Autodesk Inventor part; units mm, degrees
ref_plane "Work Plane1" through (-65, 0, -15) normal (0, 0, 1) x (1, 0, 0)
ref_plane "YZ Plane" through (0, 0, 0) normal (1, 0, 0) x (0, 1, 0)
ref_plane "XZ Plane" through (0, 0, 0) normal (0, 1, 0) x (-1, 0, 0)
sketch "Sketch1" plane through (0, 0, 0) normal (0, 1, 0) x (-1, 0, 0)
  line L0 (0, 0) -> (65, 0)
  line L1 (65, 0) -> (65, -30)
  line L2 (65, -30) -> (0, -30)
  line L3 (0, -30) -> (0, 0)
  dimension "d0" = 65
  dimension "d1" = 30
extrude "Extrusion1" add sketch "Sketch1" along normal blind 20
sketch "Sketch2" plane through (-65, 0, 0) normal (0, 0, 1) x (1, 0, 0)
  line L0 (5, 18) -> (15, 18)
  line L1 (15, 18) -> (15, 13)
  line L2 (15, 13) -> (5, 13)
  line L3 (5, 13) -> (5, 18)
  line L4 (0, 0) -> (65, 0)
  line L5 (30, 18) -> (30, 13)
  line L6 (30, 13) -> (20, 13)
  line L7 (20, 13) -> (20, 18)
  line L8 (20, 18) -> (30, 18)
  line L9 (45, 18) -> (45, 13)
  line L10 (45, 13) -> (35, 13)
  line L11 (35, 13) -> (35, 18)
  line L12 (35, 18) -> (45, 18)
  line L13 (60, 18) -> (60, 13)
  line L14 (60, 13) -> (50, 13)
  line L15 (50, 13) -> (50, 18)
  line L16 (50, 18) -> (60, 18)
  dimension "d4" = 10
  dimension "d5" = 5
  dimension "d6" = 13
  dimension "d7" = 5
  dimension "d10" = 15
extrude "Extrusion2" cut sketch "Sketch2" against normal blind 10
ref_plane "Work Plane1" through (-65, 0, -15) normal (0, 0, 1) x (1, 0, 0)
mirror "Mirror1" about plane through (-65, 0, -15) normal (0, 0, 1) of "Extrusion2"
properties part number "Relay"
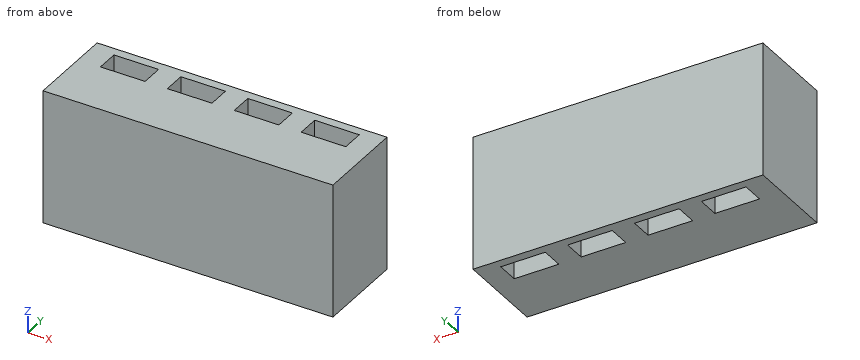
Work out the finished part from the listing and answer in its coordinate system (mm). Coordinates: 2 decimals unless noted, no trailing zeros. Order: outer loops, then holes, each group sorted by start corner. A loop starts at its lowest first (then second) coordinate and runs counter-clockwise, first axis right, second up. Notation, with made-up numbers: (-15, 56.25) - (2, 56.25) arc R5 ccw to (2, 61.25) - close; hole circle Ø8 at (22, -38.5). An arc over 180 degrees is marked (long way). Answer as a JSON object with one key per item and string values.
1. Consider line 1 (X direction, y = 17.5, z = -22); line 2 (Y direction, x = -22.5, z = -5.75); line 3 (Z direction, x = -43, y = 15). Determine where each line is inside the solid, lowest interval first.
Output values:
{"line 1": "x = -65 to -60, -50 to -45, -35 to -30, -20 to -15, -5 to 0", "line 2": "y = 0 to 13, 18 to 20", "line 3": "z = -20 to -10"}
2. Find section A-A on z = -6.75. Determine the outline of the cut face in (x, y), plus the area to 3 significant figures.
Output values:
{"outline": "(-65, 0) - (0, 0) - (0, 20) - (-65, 20) - close; hole (-60, 13) - (-50, 13) - (-50, 18) - (-60, 18) - close; hole (-45, 13) - (-35, 13) - (-35, 18) - (-45, 18) - close; hole (-30, 13) - (-20, 13) - (-20, 18) - (-30, 18) - close; hole (-15, 13) - (-5, 13) - (-5, 18) - (-15, 18) - close", "area": "1,100 mm²"}
3. Find section B-B on x = -14. Determine the outline of the cut face in (y, z).
Output values:
{"outline": "(0, -30) - (13, -30) - (13, -20) - (18, -20) - (18, -30) - (20, -30) - (20, 0) - (18, 0) - (18, -10) - (13, -10) - (13, 0) - (0, 0) - close"}
4. This flat-tipped pin is pushed along its axis until it touches: P1, Ø1.5, axis at x = -38, y = 16.5, coming from the -Z side. Where does it stop, or does it pass through?
Output values:
{"P1": "stops at z = -20"}
